```python
from build123d import *

# Parameters (mm, degrees)
EXTRUDE_1_DEPTH     = 30
SKETCH_2_R          = 1.65
CUT_EXTRUDE_1_DEPTH = 40
SKETCH_3_R          = 1.65
CUT_EXTRUDE_2_DEPTH = 40


with BuildPart() as part:
    # 草图1 → 凸台-拉伸1 (new body)
    with BuildSketch(Plane.XY):
        Polygon((0, 30), (0, 0), (30, 0), (30, 5), (5, 5), (5, 30), align=None)
    extrude(amount=EXTRUDE_1_DEPTH)

    # 草图2 → 切除-拉伸1 (cut)
    with BuildSketch(Plane(origin=(0, 5, 0), x_dir=(1, 0, 0), z_dir=(0, 1, 0))):
        with Locations(Location((23, -8, 0), (0, 0, 180))):
            Circle(SKETCH_2_R)
        with Locations(Location((23, -22, 0), (0, 0, 180))):
            Circle(SKETCH_2_R)
        with Locations(Location((12, -8, 0), (0, 0, 180))):
            Circle(SKETCH_2_R)
        with Locations(Location((12, -22, 0), (0, 0, 180))):
            Circle(SKETCH_2_R)
    extrude(amount=-CUT_EXTRUDE_1_DEPTH, mode=Mode.SUBTRACT)

    # 草图3 → 切除-拉伸2 (cut)
    with BuildSketch(Plane(origin=(5, 0, 0), x_dir=(0, 0, -1), z_dir=(1, 0, 0))):
        with Locations(Location((-22, 23, 0), (0, 0, 90))):
            Circle(SKETCH_3_R)
        with Locations(Location((-22, 12, 0), (0, 0, 90))):
            Circle(SKETCH_3_R)
        with Locations(Location((-8, 23, 0), (0, 0, 90))):
            Circle(SKETCH_3_R)
        with Locations(Location((-8, 12, 0), (0, 0, 90))):
            Circle(SKETCH_3_R)
    extrude(amount=-CUT_EXTRUDE_2_DEPTH, mode=Mode.SUBTRACT)


solid = part.part
```
The model under review builds one solid part; all positions refer to its coordinate system, in mm. A direction names the side the tool comes from. Give positions to 0.01 mm unless a question says otherwise; leave off trailing zeros. Order: outer loops, then holes, each group sorted by start corner. A loop starts at its lowest first (then second) coordinate and runs counter-clockwise, first axis right, second up. Notation, with made-up numbers: (76, -6) - (83, -6) arc R23 ccw to (83, 19) - close; hole circle Ø4 at (0, 66). An arc over 180 degrees is marked (long way). Use CSV: the item, a comma, the result in double quotes. Start each with the question number.
Q1. We need section B-B, the plane x = 23. Write out the cut boundary in (y, z).
Q2. To check wall thickness, follow line 1 along Z through (x, y) = (12, 2.85); line 2 along Y through (x, z) = (2.5, 21.5); line 3 along X through (y, z) = (1.5, 7). State the ranges of each line that lie inside material, in increasing order. Write a range as [from, to].
Q3. The part is to be moulded in two halves that separate along Z. For faces 1 (the flat face through (0, 15, 15)), 2 (the flat face through (4, 10, 0)), 3 (the cylindrical face through (10.426, 2.535, 8.496)), say which applies: +Z half, -Z half, draft (parallel to the pull), parting line (faces both ways), or undercut.
Q4. We need section D-D, the plane y = 4.5. Write out the cut boundary in (x, z), and give its area (3 significant figures).
Q5. Clearance check with flat-ended pins moving along their axes: pin 1 Ø4 at (y, z) = (27, 17.5) entering from +X; pin 2 Ø6 at (x, z) = (24.5, 24) entering from +Y. State where each tip first meets the part, or that it passes through.
Q6. We need section A-A, the plane z = 22. Write out the cut boundary in (x, y), and give its area (3 significant figures).
Q7. Tool access review of faces 4 (the flat face through (18, 5, 15)), 5 (the flat face through (3, 30, 15)): name each direction out of +Z, -Z, +X, -X, +Y, -Y from which nothing blocks a thin tool from reaching the whole face with its end or side.
Outcome:
1,outline,"(0, 0) - (5, 0) - (5, 6.35) - (0, 6.35) - close; (0, 9.65) - (5, 9.65) - (5, 20.35) - (0, 20.35) - close; (0, 23.65) - (5, 23.65) - (5, 30) - (0, 30) - close"
2,line 1,"z = [0, 6.35], [9.65, 20.35], [23.65, 30]"
2,line 2,"y = [0, 10.43], [13.57, 21.43], [24.57, 30]"
2,line 3,"x = [0, 10.69], [13.31, 21.69], [24.31, 30]"
3,face 1,"draft"
3,face 2,"-Z half"
3,face 3,"undercut"
4,outline,"(0, 0) - (30, 0) - (30, 30) - (0, 30) - close; hole circle Ø3.3 at (12, 8); hole circle Ø3.3 at (12, 22); hole circle Ø3.3 at (23, 8); hole circle Ø3.3 at (23, 22)"
4,area,"866 mm^2"
5,pin 1,"stops at x = 5"
5,pin 2,"stops at y = 5"
6,outline,"(0, 0) - (10.35, 0) - (10.35, 5) - (5, 5) - (5, 10.35) - (0, 10.35) - close; (0, 13.65) - (5, 13.65) - (5, 21.35) - (0, 21.35) - close; (0, 24.65) - (5, 24.65) - (5, 30) - (0, 30) - close; (13.65, 0) - (21.35, 0) - (21.35, 5) - (13.65, 5) - close; (24.65, 0) - (30, 0) - (30, 5) - (24.65, 5) - close"
6,area,"209 mm^2"
7,face 4,"+Z, -Z, +X, +Y"
7,face 5,"+Z, -Z, +X, -X, +Y"
